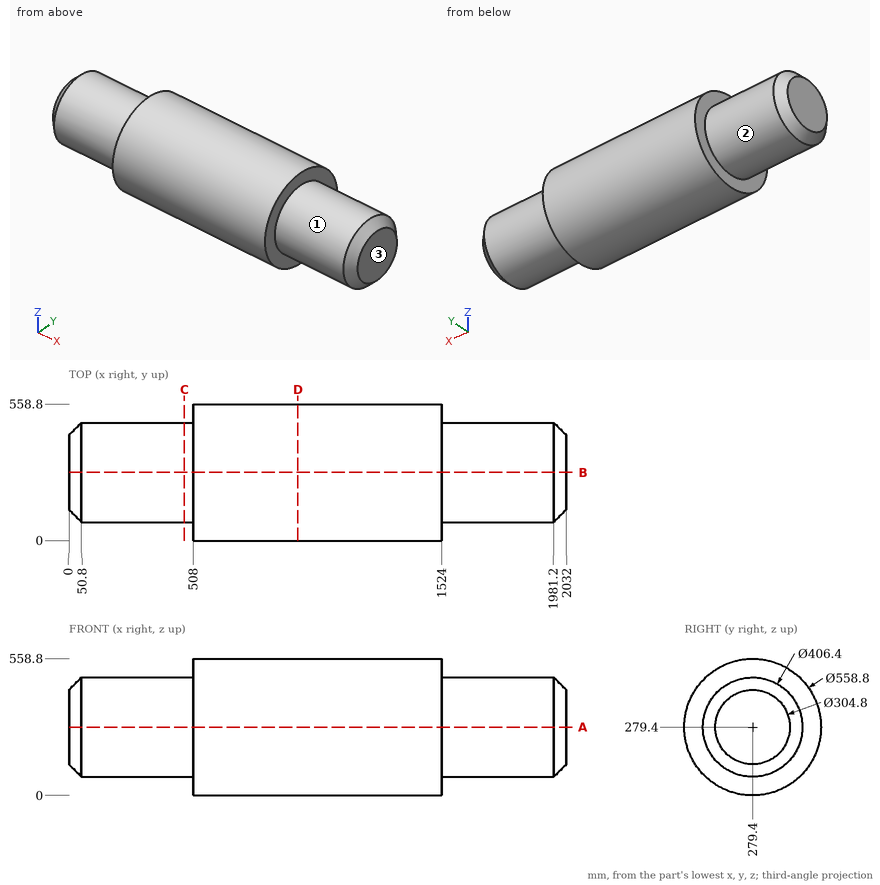
Job drawing, mm, ordinate dimensions from the low corner. One solid piece. A direction names the side the tool comes from. Round coordinates to 2 decimals unless told otherwise and drop trailing zeros. Loops run counter-clockwise (first coordinate to the right, second up) from the corner with the lowest first, then second, coordinate; pieces in that order, holes last.
Item 1: Drop flat-ended pins along their axis: P1, Ø5, axis at y = 125, z = 360.5, coming from the -X side; P2, Ø1.5, axis at x = 1225.5, z = 387.5, coming from the +Y side; P3, Ø1, axis at x = 827, z = 246, coming from the -Y side. Give the stop position or say it passes through.
Item 2: 3-axis set-ups, long thin cutter, end or side, ignore diameter. For the marked faces 1, 2 and 3: which of +Z, -Z, +X, -X, +Y, -Y reach the whole face in a straight line?
Item 3: Cut at C-C, the plane x = 471.5. Give the cut face in (y, z).
Item 4: Cut at A-A, the plane z = 279.4. Give the cut face in (x, y).
Item 5: Cut at D-D, the plane x = 935.5. Give the cut face in (y, z).
Item 6: Drill centre lines: line 1 (X direction, y = 309, z = 498.5); line 2 (Y direction, x = 1169.5, z = 268.5); line 3 (Y direction, x = 368, z = 270). Where is each one in solid material? Low to high.
A:
1. P1: stops at x = 19.5
1. P2: stops at y = 537.35
1. P3: stops at y = 1.94
2. face 1: +X
2. face 2: -X
2. face 3: +Z, -Z, +X, +Y, -Y
3. outline: circle Ø406.4 at (279.4, 279.4)
4. outline: (0, 127) - (50.8, 76.2) - (508, 76.2) - (508, 0) - (1524, 0) - (1524, 76.2) - (1981.2, 76.2) - (2032, 127) - (2032, 431.8) - (1981.2, 482.6) - (1524, 482.6) - (1524, 558.8) - (508, 558.8) - (508, 482.6) - (50.8, 482.6) - (0, 431.8) - close
5. outline: circle Ø558.8 at (279.4, 279.4)
6. line 1: x = 508 to 1524
6. line 2: y = 0.21 to 558.59
6. line 3: y = 76.42 to 482.38
